Autodesk Inventor part; units mm, degrees
ref_plane "YZ Plane" through (0, 0, 0) normal (1, 0, 0) x (0, 1, 0)
ref_plane "XZ Plane" through (0, 0, 0) normal (0, 1, 0) x (-1, 0, 0)
ref_plane "XY Plane" through (0, 0, 0) normal (0, 0, 1) x (1, 0, 0)
sketch "Náčrt1" plane through (0, 0, 0) normal (0, 1, 0) x (-1, 0, 0)
  line L0 (0, 0) -> (18, 0)
  line L1 (18, 0) -> (18, -30)
  line L2 (18, -30) -> (0, -30)
  line L3 (0, -30) -> (0, 0)
  circle A0 centre (11, -5) radius 3
  circle A1 centre (11, -25) radius 3
  dimension "d0" = 18
  dimension "d1" = 30
  dimension "d2" = 6
  dimension "d3" = 6
  dimension "d4" = 11
  dimension "d5" = 11
  dimension "d6" = 5
  dimension "d7" = 5
extrude "Vysunutí1" add sketch "Náčrt1" along normal blind 3
equation "\"d5\" = d4"
equation "\"d7\" = d6"
properties part number "prilozka"
Could you check a few things on this model? Use its own coordinates, in mm. Round coordinates to 2 decimals unless told otherwise and drop trailing zeros. Loops run counter-clockwise (first coordinate to the right, second up) from the corner with the lowest first, then second, coordinate; pieces in that order, holes last. Notation, with made-up numbers: (-24, -7) - (-19, -7) arc R24 cw to (-19, 19) - close; hole circle Ø1 at (23.5, 12). An arc over 180 degrees is marked (long way). Answer as CSV lines item,"result".
1. I want a section at A-A on x = -11. List the corners of the cut face in (y, z) for me.
Filled in:
outline,"(0, -30) - (3, -30) - (3, -28) - (0, -28) - close; (0, -22) - (3, -22) - (3, -8) - (0, -8) - close; (0, -2) - (3, -2) - (3, 0) - (0, 0) - close"
2. We'd pull the mould along Z, two halves only. Please class faces 1 (the face through (-9, 1, 0)), 2 (the face through (-8.6, 1.5, -23.2)), 3 (the face through (-9, 1, -30)), 4 (the face through (-18, 1, -15)): +Z half, -Z half, draft (parallel to the pull), parting line (faces both ways), or undercut.
Filled in:
face 1,"+Z half"
face 2,"undercut"
face 3,"-Z half"
face 4,"draft"
3. I want a section at D-D on z = -6. List the corners of the cut face in (x, y) for me.
Filled in:
outline,"(-18, 0) - (-13.83, 0) - (-13.83, 3) - (-18, 3) - close; (-8.17, 0) - (0, 0) - (0, 3) - (-8.17, 3) - close"
4. Please list where these lines run through material, in increasing order: line 1 along Z through (x, y) = (-11, 0.65); line 2 along Z through (x, y) = (-13.75, 2.65); line 3 along X through (y, z) = (2.7, -27). Write a range as [from, to].
Filled in:
line 1,"z = [-30, -28], [-22, -8], [-2, 0]"
line 2,"z = [-30, -26.2], [-23.8, -6.2], [-3.8, 0]"
line 3,"x = [-18, -13.24], [-8.76, 0]"
5. I want a section at C-C on y = 1.15. List the corners of the cut face in (x, z) for me.
Filled in:
outline,"(-18, -30) - (0, -30) - (0, 0) - (-18, 0) - close; hole circle Ø6 at (-11, -25); hole circle Ø6 at (-11, -5)"
6. I want a section at B-B on z = -25. List the corners of the cut face in (x, y) for me.
Filled in:
outline,"(-18, 0) - (-14, 0) - (-14, 3) - (-18, 3) - close; (-8, 0) - (0, 0) - (0, 3) - (-8, 3) - close"
